from build123d import *

# Parameters (mm, degrees)
BOSS_EXTRUDE1_DEPTH = 2
SKETCH2_W           = 2
SKETCH2_H           = 20
CUT_EXTRUDE1_DEPTH  = 10
SKETCH3_W           = 20
SKETCH3_H           = 2
BOSS_EXTRUDE2_DEPTH = 2


with BuildPart() as part:
    # Sketch1 → Boss-Extrude1 (new body)
    with BuildSketch(Plane(origin=(0, 0, 0), x_dir=(0, 0, -1), z_dir=(1, 0, 0))):
        Polygon((-97, -35), (97, -35), (97, 0), (99, 0), (99, 20), (97, 20), (97, 35), (-97, 35), (-97, 20), (-99, 20), (-99, 0), (-97, 0), align=None)
    extrude(amount=BOSS_EXTRUDE1_DEPTH)

    # Sketch2 → Cut-Extrude1 (cut)
    with BuildSketch(Plane(origin=(2, 0, 0), x_dir=(0, 0, -1), z_dir=(1, 0, 0))):
        with Locations((-98, 10)):
            Rectangle(SKETCH2_W, SKETCH2_H)
        with Locations((98, 10)):
            Rectangle(SKETCH2_W, SKETCH2_H)
    extrude(amount=-CUT_EXTRUDE1_DEPTH, mode=Mode.SUBTRACT)

    # Sketch3 → Boss-Extrude2 (add)
    with BuildSketch(Plane(origin=(2, 0, 0), x_dir=(0, 0, -1), z_dir=(1, 0, 0))):
        with Locations((-67, -36)):
            Rectangle(SKETCH3_W, SKETCH3_H)
        with Locations((-27, -36)):
            Rectangle(SKETCH3_W, SKETCH3_H)
        with Locations((27, -36)):
            Rectangle(SKETCH3_W, SKETCH3_H)
        with Locations((67, -36)):
            Rectangle(SKETCH3_W, SKETCH3_H)
    extrude(amount=-BOSS_EXTRUDE2_DEPTH)


solid = part.part
Part model, mm, in its own coordinate system. Give positions to 0.01 mm unless a question says otherwise; leave off trailing zeros. Order: outer loops, then holes, each group sorted by start corner. A loop starts at its lowest first (then second) coordinate and runs counter-clockwise, first axis right, second up. Notation, with made-up numbers: (-1.75, 23.5) -> (23.25, 23.5) arc R20 cw to (23.25, 27.5) -> close; hole circle Ø3 at (-26.75, 63). An arc over 180 degrees is marked (long way). Use one line per item in the form item = value.
(1) Saw through at A-A (x = 1.6). Write the cut outline in (y, z).
Solution:
outline = (-37, -77) -> (-35, -77) -> (-35, -97) -> (35, -97) -> (35, 97) -> (-35, 97) -> (-35, 77) -> (-37, 77) -> (-37, 57) -> (-35, 57) -> (-35, 37) -> (-37, 37) -> (-37, 17) -> (-35, 17) -> (-35, -17) -> (-37, -17) -> (-37, -37) -> (-35, -37) -> (-35, -57) -> (-37, -57) -> close
(2) Flat gauge pins, fed straight in: P1, Ø1, axis at x = 0.5, z = 5, coming from the -Y side; P2, Ø0.6, axis at x = 1.5, y = -36, coming from the +Z side; P3, Ø0.6, axis at x = 1.5, y = -36, coming from the -Z side. Where does each tip first touch, or does it go through?
Solution:
P1 = -35
P2 = 77
P3 = -77
(3) Drill centre line: line 1 (Y direction, x = 1.45, z = 80). Where is it in solid material? Low to high. Write a range as from..to.
Solution:
line_1 = -35..35
(4) Saw through at B-B (z = 8). Write the cut outline in (x, y), then the cut area to 3 significant figures.
Solution:
outline = (0, -35) -> (2, -35) -> (2, 35) -> (0, 35) -> close
area = 140 mm²
